Part model, mm, in its own coordinate system. A direction names the side the tool comes from. Give positions to 0.01 mm unless a question says otherwise; leave off trailing zeros. Order: outer loops, then holes, each group sorted by start corner. A loop starts at its lowest first (then second) coordinate and runs counter-clockwise, first axis right, second up. Notation, with made-up numbers: (82.5, 23) -> (104.5, 23) arc R25 ccw to (104.5, 40) -> close; hole circle Ø9 at (-29.5, 33). An arc over 180 degrees is marked (long way). Write item = value, one per line. Start each with the question number.
(1) Saw through at D-D, the plane z = 10. List the corners of the cut face in (x, y).
(2) Saw through at C-C, the plane x = -7.5. List the corners of the cut face in (y, z).
(3) Flat gauge pins, fed straight in: pin 1 (3.5 mm diameter, centred on x = -15, z = 66.1, fed in from +Y); pin 2 (1.5 mm diameter, centred on x = -2.5, z = 41.5, fed in from -Y). Where does each tip first touch, or does it go through?
(4) Two-plate mould, pull along Y, no slides. Class faces 1 (the flat face through (15, 15, 45)), 2 (the flat face through (-5, 13, 47)), 3 (the flat face through (-10.25, -6, 47)): pulls with the +Y half, pulls with the -Y half, needs draft (parallel to the pull), parting line crosses it, or undercut.
(5) Which spindle directions (+Z, -Z, +X, -X, +Y, -Y) get a long thin tool onto all of the face, cutting with end or side? Do faces 4 (the flat face through (0, -2.45, 47)), 5 (the flat face through (-5.25, -13, 47)), 6 (the flat face through (10, 13, 47)), 7 (the flat face through (15, 5, 66)). Say none if no direction does.
(6) Saw through at B-B, the plane y = -7.75. List the corners of the cut face in (x, z).
(7) Probe line 1 along X through (y, z) = (13.25, 80); line 2 along Z through (x, y) = (15, 10.5); line 3 along X through (y, z) = (7.25, 66.1). List the from-to ranges inside material, lowest first. Write a range as from..to.
(8) Saw through at A-A, the plane y = 11. List the corners of the cut face in (x, z).
from build123d import *

# Parameters (mm, degrees)
CROQUIS1_W              = 40
CROQUIS1_H              = 30
SALIENTE_EXTRUIR1_DEPTH = 92.2
CORTAR_EXTRUIR1_DEPTH   = 96.529262532
CROQUIS3_W              = 5
CROQUIS3_H              = 92.2
CORTAR_EXTRUIR2_DEPTH   = 5
CROQUIS4_R              = 2
CORTAR_EXTRUIR3_DEPTH   = 10


with BuildPart() as part:
    # Croquis1 → Saliente-Extruir1 (new body)
    with BuildSketch(Plane.XY):
        Rectangle(CROQUIS1_W, CROQUIS1_H)
    extrude(amount=SALIENTE_EXTRUIR1_DEPTH)

    # Croquis2 → Cortar-Extruir1 (cut, through all)
    with BuildSketch(Plane.XY.offset(92.2)):
        Polygon((-10.25, -2.45), (-10.25, -10.2), (-5.25, -10.2), (-5.25, -15), (5.25, -15), (5.25, -10.2), (10.25, -10.2), (10.25, -2.45), align=None)
    extrude(amount=-CORTAR_EXTRUIR1_DEPTH, mode=Mode.SUBTRACT)

    # Croquis3 → Cortar-Extruir2 (cut)
    with BuildSketch(Plane(origin=(0, 15, 0), x_dir=(1, 0, 0), z_dir=(0, 1, 0))):
        with Locations((-7.5, -46.1)):
            Rectangle(CROQUIS3_W, CROQUIS3_H)
        with Locations((7.5, -46.1)):
            Rectangle(CROQUIS3_W, CROQUIS3_H)
    extrude(amount=-CORTAR_EXTRUIR2_DEPTH, mode=Mode.SUBTRACT)

    # Croquis4 → Cortar-Extruir3 (cut)
    with BuildSketch(Plane(origin=(0, 15, 0), x_dir=(1, 0, 0), z_dir=(0, 1, 0))):
        with Locations(Location((-15, -26.1, 0), (0, 0, 270))):
            Circle(CROQUIS4_R)
        with Locations(Location((-15, -66.1, 0), (0, 0, 270))):
            Circle(CROQUIS4_R)
        with Locations(Location((15, -66.1, 0), (0, 0, 90))):
            Circle(CROQUIS4_R)
        with Locations(Location((15, -26.1, 0), (0, 0, 90))):
            Circle(CROQUIS4_R)
    extrude(amount=-CORTAR_EXTRUIR3_DEPTH, mode=Mode.SUBTRACT)


solid = part.part
Results list:
q1.outline = (-20, -15) -> (-5.25, -15) -> (-5.25, -10.2) -> (-10.25, -10.2) -> (-10.25, -2.45) -> (10.25, -2.45) -> (10.25, -10.2) -> (5.25, -10.2) -> (5.25, -15) -> (20, -15) -> (20, 15) -> (10, 15) -> (10, 10) -> (5, 10) -> (5, 15) -> (-5, 15) -> (-5, 10) -> (-10, 10) -> (-10, 15) -> (-20, 15) -> close
q2.outline = (-15, 0) -> (-10.2, 0) -> (-10.2, 92.2) -> (-15, 92.2) -> close; (-2.45, 0) -> (10, 0) -> (10, 92.2) -> (-2.45, 92.2) -> close
q3.pin_1 = 5
q3.pin_2 = -2.45
q4.face_1 = pulls with the +Y half
q4.face_2 = needs draft
q4.face_3 = undercut
q5.face_4 = +Z, -Z
q5.face_5 = +Z, -Z, -Y
q5.face_6 = +Z, -Z, +Y
q5.face_7 = +Y
q6.outline = (-20, 0) -> (-10.25, 0) -> (-10.25, 92.2) -> (-20, 92.2) -> close; (10.25, 0) -> (20, 0) -> (20, 92.2) -> (10.25, 92.2) -> close
q7.line_1 = -20..-10, -5..5, 10..20
q7.line_2 = 0..24.1, 28.1..64.1, 68.1..92.2
q7.line_3 = -20..-17, -13..13, 17..20
q8.outline = (-20, 0) -> (-10, 0) -> (-10, 92.2) -> (-20, 92.2) -> close; (-5, 0) -> (5, 0) -> (5, 92.2) -> (-5, 92.2) -> close; (10, 0) -> (20, 0) -> (20, 92.2) -> (10, 92.2) -> close; hole circle Ø4 at (-15, 26.1); hole circle Ø4 at (-15, 66.1); hole circle Ø4 at (15, 26.1); hole circle Ø4 at (15, 66.1)
